```python
from build123d import *

# Parameters (mm, degrees)
SKETCH_1_R          = 15
SKETCH_1_R_2        = 2.5
EXTRUDE_1_DEPTH     = 5
SKETCH_2_W          = 2
SKETCH_2_H          = 1
CUT_EXTRUDE_1_DEPTH = 10
SKETCH_3_R          = 10
CUT_EXTRUDE_2_DEPTH = 10
CUT_EXTRUDE_3_DEPTH = 10


with BuildPart() as part:
    # 草图1 → 凸台-拉伸1 (new body)
    with BuildSketch(Plane(origin=(0, 0, 0), x_dir=(1, 0, 0), z_dir=(0, 1, 0))):
        with Locations(Location((0, 0, 0), (0, 0, 270))):
            Circle(SKETCH_1_R)
        with Locations(Location((0, 0, 0), (0, 0, 270))):
            Circle(SKETCH_1_R_2, mode=Mode.SUBTRACT)
    extrude(amount=EXTRUDE_1_DEPTH)

    # 草图2 → 切除-拉伸1 (cut)
    with BuildSketch(Plane(origin=(0, 5, 0), x_dir=(1, 0, 0), z_dir=(0, 1, 0))):
        with Locations((0, 2.5)):
            Rectangle(SKETCH_2_W, SKETCH_2_H)
    extrude(amount=-CUT_EXTRUDE_1_DEPTH, mode=Mode.SUBTRACT)

    # 草图3 → 切除-拉伸2 (cut)
    with BuildSketch(Plane(origin=(0, 5, 0), x_dir=(1, 0, 0), z_dir=(0, 1, 0))):
        with Locations((0, 20)):
            Circle(SKETCH_3_R)
        with Locations((20, 0)):
            Circle(SKETCH_3_R)
        with Locations((0, -20)):
            Circle(SKETCH_3_R)
        with Locations((-20, 0)):
            Circle(SKETCH_3_R)
    extrude(amount=-CUT_EXTRUDE_2_DEPTH, mode=Mode.SUBTRACT)

    # 草图4 → 切除-拉伸3 (cut)
    with BuildSketch(Plane(origin=(0, 5, 0), x_dir=(1, 0, 0), z_dir=(0, 1, 0))):
        with BuildLine():
            Line((-12.639931989, 9.104398083), (-7.424621202, 3.889087297))
            ThreePointArc((-7.424621202, 3.889087297), (-3.889087297, 3.889087297), (-3.889087297, 7.424621202))
            Line((-3.889087297, 7.424621202), (-9.104398083, 12.639931989))
            Line((-9.104398083, 12.639931989), (-12.639931989, 9.104398083))
        make_face()
        with BuildLine():
            Line((12.639931989, 9.104398083), (7.424621202, 3.889087297))
            ThreePointArc((7.424621202, 3.889087297), (3.889087297, 3.889087297), (3.889087297, 7.424621202))
            Line((3.889087297, 7.424621202), (9.104398083, 12.639931989))
            Line((9.104398083, 12.639931989), (12.639931989, 9.104398083))
        make_face()
        with BuildLine():
            Line((9.104398083, -12.639931989), (3.889087297, -7.424621202))
            ThreePointArc((3.889087297, -7.424621202), (3.889087297, -3.889087297), (7.424621202, -3.889087297))
            Line((7.424621202, -3.889087297), (12.639931989, -9.104398083))
            Line((12.639931989, -9.104398083), (9.104398083, -12.639931989))
        make_face()
        with BuildLine():
            Line((-12.639931989, -9.104398083), (-7.424621202, -3.889087297))
            ThreePointArc((-7.424621202, -3.889087297), (-3.889087297, -3.889087297), (-3.889087297, -7.424621202))
            Line((-3.889087297, -7.424621202), (-9.104398083, -12.639931989))
            Line((-9.104398083, -12.639931989), (-12.639931989, -9.104398083))
        make_face()
    extrude(amount=-CUT_EXTRUDE_3_DEPTH, mode=Mode.SUBTRACT)


solid = part.part
```
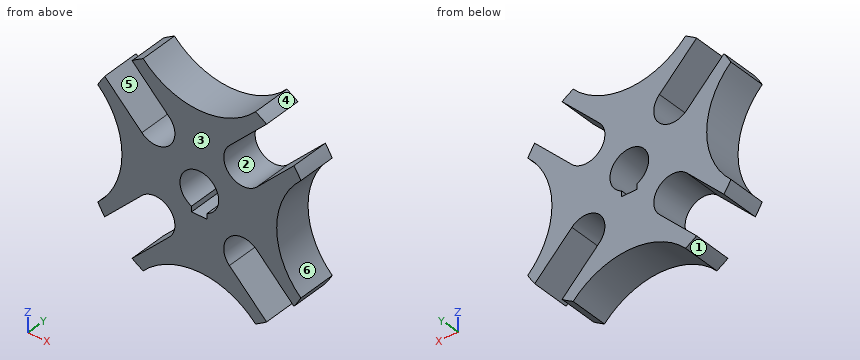
Part model, mm, in its own coordinate system. Face numbers are marked on the shaded views. A direction names the side the tool comes from. Give positions to 0.01 mm unless a question says otherwise; leave off trailing zeros. Order: outer loops, then holes, each group sorted by start corner. A loop starts at its lowest first (then second) coordinate and runs counter-clockwise, first axis right, second up. Notation, with made-up numbers: M -9,15.25 L 30,15.25 A16 cw 30,33.25 Z; hole C 2.5,27.25 d3. An arc over 180 degrees is marked long. Use a Markdown table: item, result. Add a question column.
(1) Saw through at B-B, the plane x = 0. Give the cut face in (y, z).
(2) Saw through at A-A, the plane z = 0. Give the cut face in (x, y), and give its area (3 significant figures).
(3) Drop flat-ended pins along their axis: P1, Ø1, axis at x = 1.5, y = 2, coming from the +Z side; P2, Ø1, axis at x = 0.5, y = 2.5, coming from the +Z side; P3, Ø3, axis at x = 2.5, y = 1, coming from the -Z side; P4, Ø6, axis at x = -8.5, z = 2, coming from the -Y side. Give the stop position or say it passes through.
(4) Mould opens along X. For the marked faces 1, 2, 3 and 4 say: +X half, -X half, draft (parallel to the pull), parting line (faces both ways), or undercut.
(5) 3-axis set-ups, long thin cutter, end or side, ignore diameter. For the marked faces 5 and 6: which of +Z, -Z, +X, -X, +Y, -Y reach the whole face in a straight line?
(6) Probe line 1 along Z through (x, y) = (0, 2.1); line 2 along X through (y, z) = (1.85, 8.25); line 3 along X through (y, z) = (1.9, -7.25). List the from-to ranges inside material, lowest first. Write a range as [from, to].
(7) Saw through at C-C, the plane y = 1.45. Give the cut face in (x, z) (3 decimals), and give its area (3 significant figures).
(8) Saw through at D-D, the plane z = -7.75. Give the cut face in (x, y), and give its area (3 significant figures).
Answer key:
| question | item | result |
|---|---|---|
| 1 | outline | M 0,-10 L 5,-10 L 5,-3 L 0,-3 Z; M 0,2.5 L 5,2.5 L 5,10 L 0,10 Z |
| 2 | outline | M -10,0 L -2.5,0 L -2.5,5 L -10,5 Z; M 2.5,0 L 10,0 L 10,5 L 2.5,5 Z |
| 2 | area | 75.0 mm^2 |
| 3 | P1 | z = 10.2 |
| 3 | P2 | z = 10.05 |
| 3 | P3 | z = -10.83 |
| 3 | P4 | y = 0 |
| 4 | face 1 | -X half |
| 4 | face 2 | undercut |
| 4 | face 3 | draft |
| 4 | face 4 | +X half |
| 5 | face 5 | +Y, -Y |
| 5 | face 6 | +X, +Y, -Y |
| 6 | line 1 | [-10, -3], [2.5, 10] |
| 6 | line 2 | [-12.53, -11.79], [-4.71, 4.71], [11.79, 12.53] |
| 6 | line 3 | [-13.11, -10.79], [-3.73, 3.73], [10.79, 13.11] |
| 7 | outline | M -13.125,-7.262 A15 ccw -12.226,-8.69 L -7.425,-3.889 A2.5 cw -3.889,-7.425 L -8.69,-12.226 A15 ccw -7.262,-13.125 A10 cw 7.262,-13.125 A15 ccw 8.69,-12.226 L 3.889,-7.425 A2.5 cw 7.425,-3.889 L 12.226,-8.69 A15 ccw 13.125,-7.262 A10 cw 13.125,7.262 A15 ccw 12.226,8.69 L 7.425,3.889 A2.5 cw 3.889,7.425 L 8.69,12.226 A15 ccw 7.262,13.125 A10 cw -7.262,13.125 A15 ccw -8.69,12.226 L -3.889,7.425 A2.5 cw -7.425,3.889 L -12.226,8.69 A15 ccw -13.125,7.262 A10 cw Z; hole M -1,-3 L 1,-3 L 1,-2.291 A2.5 ccw long -1,-2.291 Z |
| 7 | area | 309 mm^2 |
| 8 | outline | M -12.84,0 L -11.29,0 L -11.29,5 L -12.84,5 Z; M -4.21,0 L 4.21,0 L 4.21,5 L -4.21,5 Z; M 11.29,0 L 12.84,0 L 12.84,5 L 11.29,5 Z |
| 8 | area | 57.7 mm^2 |
